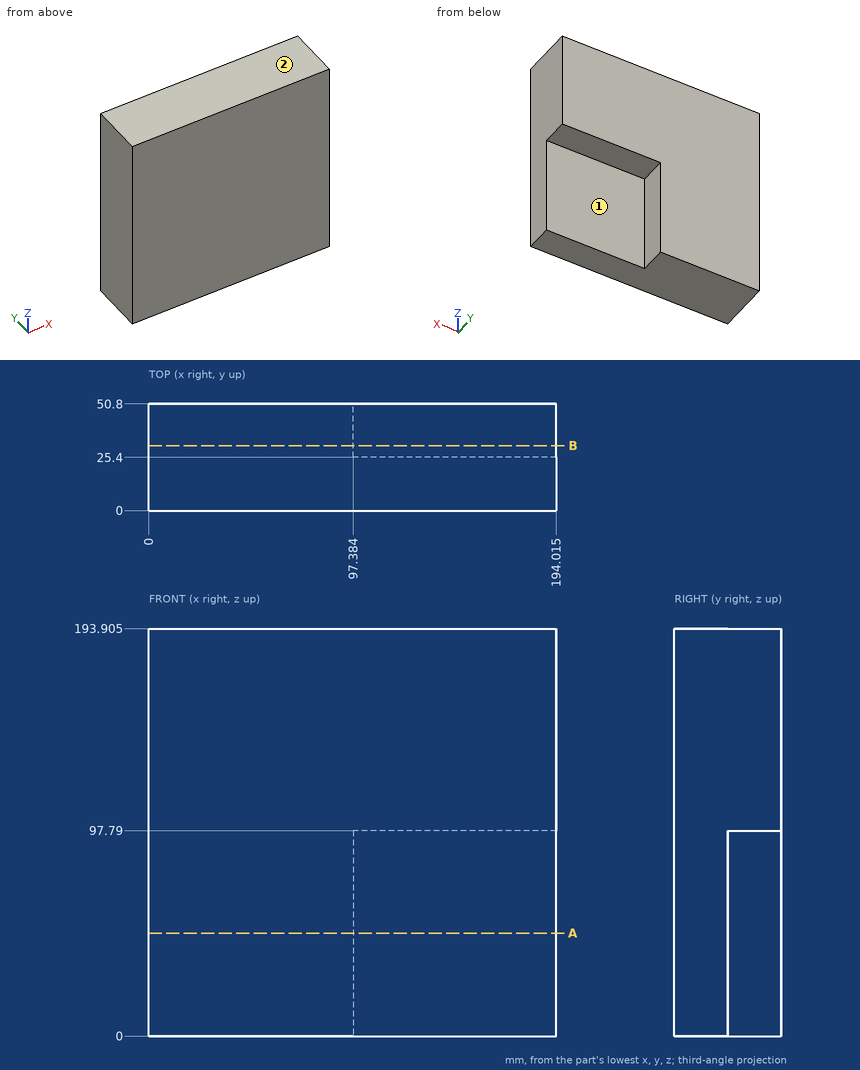
Answer from the drawing. Dimensions are ordinates in mm from the lowest x, y and z of the part. A direction names the side the tool comes from. Round coordinates to 2 decimals unless told otherwise and drop trailing zeros. Order: outer loops, then holes, each group sorted by start corner. A loop starts at its lowest first (then second) coordinate and runs counter-clockwise, first axis right, second up.
1) Flat-ended cylindrical pins translate along their axes: pin 1 (12 mm diameter, centred on y = 29, z = 62, fed in from +X) (3 decimals); pin 2 (5 mm diameter, centred on x = 147.5, z = 39.5, fed in from +Y); pin 3 (2 mm diameter, centred on y = 29.5, z = 75, fed in from +X); pin 4 (7.5 mm diameter, centred on x = 148, y = 32, fed in from -Z). Find the tip coordinate at first contact, or state that the pin passes through.
2) For the marked faces 1 and 2, determine the directions among +Z, -Z, +X, -X, +Y, -Y from which every point of the face is accessible in a straight line to the end or side of a thin tool.
3) The part is cut by section A-A on z = 49. Write down the section's boundary in (x, y) (1 decimal).
4) The part is cut by section B-B on y = 31. Write down the section's boundary in (x, z) (1 decimal), plus the area to 3 significant figures.
5) Straight lines are drawn through the part: L1, parallel to X at y = 39.5, z = 80; L2, parallel to Y at x = 177.5, z = 61.5; L3, parallel to Z at x = 139, y = 36.5 (1 decimal). For each, find the intervals that lie inside material, in ascending order.
Resolved:
1. pin 1: stops at x = 194.015
1. pin 2: stops at y = 25.4
1. pin 3: stops at x = 97.38
1. pin 4: stops at z = 97.79
2. face 1: -Z, +X, +Y
2. face 2: +Z, +X, -X, +Y, -Y
3. outline: (0, 0) - (194, 0) - (194, 25.4) - (97.4, 25.4) - (97.4, 50.8) - (0, 50.8) - close
4. outline: (0, 0) - (97.4, 0) - (97.4, 97.8) - (194, 97.8) - (194, 193.9) - (0, 193.9) - close
4. area: 28,200 mm2
5. L1: x = 0 to 97.38
5. L2: y = 0 to 25.4
5. L3: z = 97.8 to 193.9
